```python
from build123d import *

# Parameters (mm, degrees)
SKETCH_1_R          = 33.5
EXTRUDE_1_DEPTH     = 25.5
SKETCH_2_R          = 23
CUT_EXTRUDE_1_DEPTH = 23.5
SKETCH_3_R          = 5.75
EXTRUDE_2_DEPTH     = 26
CUT_EXTRUDE_2_DEPTH = 20


with BuildPart() as part:
    # Эскиз1 → Бобышка-Вытянуть1 (new body)
    with BuildSketch(Plane(origin=(0, 0, 0), x_dir=(1, 0, 0), z_dir=(0, 1, 0))):
        with Locations(Location((0, 0, 0), (0, 0, 270))):
            Circle(SKETCH_1_R)
    extrude(amount=EXTRUDE_1_DEPTH)

    # Эскиз2 → Вырез-Вытянуть1 (cut)
    with BuildSketch(Plane(origin=(0, 25.5, 0), x_dir=(1, 0, 0), z_dir=(0, 1, 0))):
        with Locations(Location((0, 0, 0), (0, 0, 270))):
            Circle(SKETCH_2_R)
    extrude(amount=-CUT_EXTRUDE_1_DEPTH, mode=Mode.SUBTRACT)

    # Эскиз3 → Бобышка-Вытянуть2 (add)
    with BuildSketch(Plane(origin=(0, 2, 0), x_dir=(1, 0, 0), z_dir=(0, 1, 0))):
        with Locations(Location((0, 0, 0), (0, 0, 90))):
            Circle(SKETCH_3_R)
    extrude(amount=EXTRUDE_2_DEPTH)

    # Эскиз4 → Вырез-Вытянуть2 (cut)
    with BuildSketch(Plane(origin=(0, 28, 0), x_dir=(1, 0, 0), z_dir=(0, 1, 0))):
        with BuildLine():
            Line((2.436698586, 1.75), (-2.436698586, 1.75))
            ThreePointArc((-2.436698586, 1.75), (-3, 0), (-2.436698586, -1.75))
            Line((-2.436698586, -1.75), (2.436698586, -1.75))
            ThreePointArc((2.436698586, -1.75), (2.855704445, -0.919212772), (3, 0))
            ThreePointArc((3, 0), (2.855704445, 0.919212772), (2.436698586, 1.75))
        make_face()
    extrude(amount=-CUT_EXTRUDE_2_DEPTH, mode=Mode.SUBTRACT)


solid = part.part
```
Input: part model. Units: mm. Frame: model coordinates. A direction names the side the tool comes from. Coordinates: 2 decimals unless noted, no trailing zeros. Loops run counter-clockwise (first coordinate to the right, second up) from the corner with the lowest first, then second, coordinate; pieces in that order, holes last. Notation, with made-up numbers: (-3, 10) - (22, 10) arc R31 ccw to (22, 48) - close; hole circle Ø5 at (18.5, 57.25). An arc over 180 degrees is marked (long way). Answer in a Markdown table with one row per item.
(1) Cut plane B-B on x = -9. Output: boundary loops of the cut face in (y, z), plus the area to 3 significant figures.
Model answer:
| item | result |
|---|---|
| outline | (0, -32.27) - (25.5, -32.27) - (25.5, -21.17) - (2, -21.17) - (2, 21.17) - (25.5, 21.17) - (25.5, 32.27) - (0, 32.27) - close |
| area | 651 mm² |
(2) Set-up query: faces 1 (the face through (19.394, 13.914, 12.365)), 2 (the face through (0, 28, -2)). Return all of +Z, -Z, +X, -X, +Y, -Y with unobstructed straight access to the full face (end or side cutting, diameter ignored); none if empty.
Model answer:
| item | result |
|---|---|
| face 1 | +Y |
| face 2 | +Z, -Z, +X, -X, +Y |
(3) Cut plane A-A on y = 15. Output: boundary loops of the cut face in (x, z).
Model answer:
| item | result |
|---|---|
| outline | circle Ø67 at (0, 0); circle Ø11.5 at (0, 0); hole circle Ø46 at (0, 0); hole (-2.44, -1.75) - (2.44, -1.75) arc R3 ccw to (2.44, 1.75) - (-2.44, 1.75) arc R3 ccw to start |
(4) Cut plane C-C on z = -22. Output: boundary loops of the cut face in (x, y).
Model answer:
| item | result |
|---|---|
| outline | (-25.26, 0) - (25.26, 0) - (25.26, 25.5) - (6.71, 25.5) - (6.71, 2) - (-6.71, 2) - (-6.71, 25.5) - (-25.26, 25.5) - close |
(5) Material intervals for L1, parallel to X at y = 12.5, z = 0; L2, parallel to Y at x = 19, z = 20.5; L3, parallel to Z at x = 17.5, y = 15, sorted ascending. Write a range as from..to.
Model answer:
| item | result |
|---|---|
| L1 | x = -33.5..-23, -5.75..-3, 3..5.75, 23..33.5 |
| L2 | y = 0..25.5 |
| L3 | z = -28.57..-14.92, 14.92..28.57 |
(6) Pin query (flat end, axial travel): P1, Ø8, axis at x = -15, z = -22, coming from the +Y side; P2, Ø1.5, axis at x = -1, y = 18, coming from the -Z side; P3, Ø3, axis at x = -11.5, z = -1.5, coming from the +Y side. Return the tip coordinate at first contact, or that it passes through.
Model answer:
| item | result |
|---|---|
| P1 | stops at y = 25.5 |
| P2 | stops at z = -33.5 |
| P3 | stops at y = 2 |
(7) Mould query, pull axis Z, two halves, no side actions, for faces 3 (the face through (-29.7, 12.6, 15.5)), 4 (the face through (0, 8, 0)), 5 (the face through (0, 0, 0)). Classes: pulls with the +Z half, pulls with the -Z half, needs draft (parallel to the pull), parting line crosses it, or undercut.
Model answer:
| item | result |
|---|---|
| face 3 | parting line crosses it |
| face 4 | undercut |
| face 5 | needs draft |
(8) Cut plane D-D on x = 4.5. Output: boundary loops of the cut face in (y, z).
Model answer:
| item | result |
|---|---|
| outline | (0, -33.2) - (25.5, -33.2) - (25.5, -22.56) - (2, -22.56) - (2, -3.58) - (28, -3.58) - (28, 3.58) - (2, 3.58) - (2, 22.56) - (25.5, 22.56) - (25.5, 33.2) - (0, 33.2) - close |
